Geometry: see drawing. Coordinates: mm, zero at the bounding-box minimum. Coordinates: 2 decimals unless noted, no trailing zeros. Order: outer loops, then holes, each group sorted by start corner. A loop starts at its lowest first (then second) coordinate and runs counter-clockwise, first axis right, second up. Notation, with made-up numbers: (5.5, -5) -> (62.5, -5) arc R23 cw to (62.5, 17) -> close; hole circle Ø7 at (-35, 70). An arc over 180 degrees is marked (long way). Use one line per item in the form item = value.
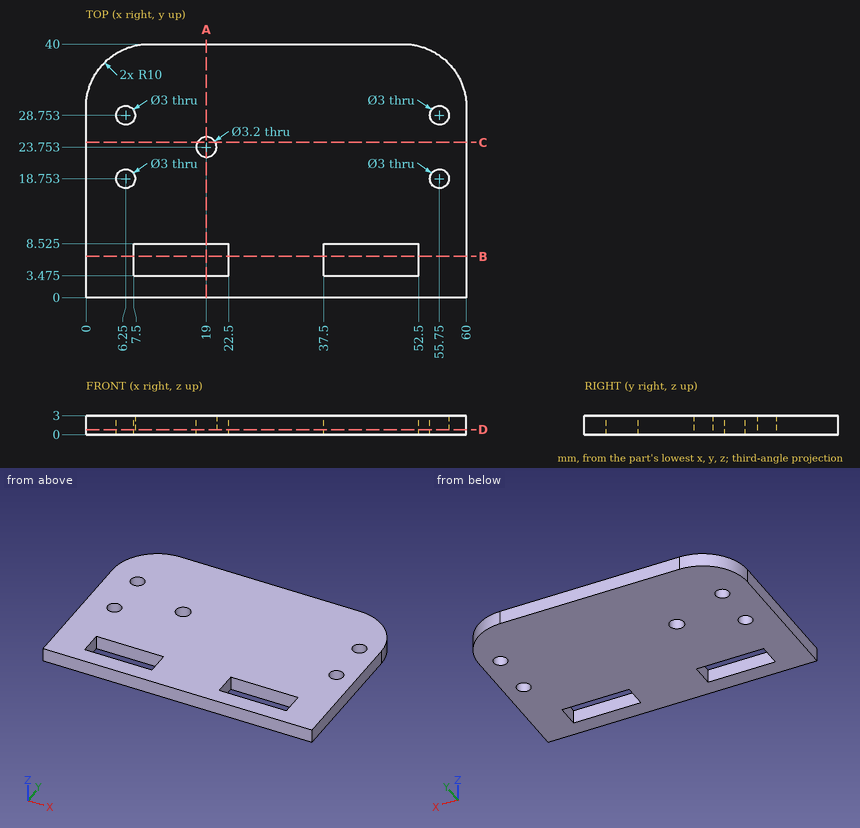
1) Section B-B, the plane y = 6.5. Output: boundary loops of the cut face in (x, z), and give its area (3 significant figures).
Results found:
outline = (0, 0) -> (7.5, 0) -> (7.5, 3) -> (0, 3) -> close; (22.5, 0) -> (37.5, 0) -> (37.5, 3) -> (22.5, 3) -> close; (52.5, 0) -> (60, 0) -> (60, 3) -> (52.5, 3) -> close
area = 90.0 mm2
2) Section C-C, the plane y = 24.5. Output: boundary loops of the cut face in (x, z) (3 decimals).
Results found:
outline = (0, 0) -> (17.585, 0) -> (17.585, 3) -> (0, 3) -> close; (20.415, 0) -> (60, 0) -> (60, 3) -> (20.415, 3) -> close
3) Contact query for flat-ended pins moving along their axis: P1, Ø0.9, axis at x = 17, z = 1, coming from the -Y side; P2, Ø2.5, axis at x = 55.75, y = 18.75, coming from the -Z side. Output: stop coordinate, or through.
Results found:
P1 = 0
P2 = through
4) Section A-A, the plane x = 19. Output: boundary loops of the cut face in (y, z) (1 decimal).
Results found:
outline = (0, 0) -> (3.5, 0) -> (3.5, 3) -> (0, 3) -> close; (8.5, 0) -> (22.2, 0) -> (22.2, 3) -> (8.5, 3) -> close; (25.4, 0) -> (40, 0) -> (40, 3) -> (25.4, 3) -> close
5) Material intervals for probe 1 along X at (y, z) = (8, 1.55); probe 2 along Y at (x, z) = (19, 0.85) (1 decimal); probe 3 along Y at (x, z) = (12, 1.9) (3 decimals), sorted ascending. Write a range as from..to.
Results found:
probe_1 = 0..7.5, 22.5..37.5, 52.5..60
probe_2 = 0..3.5, 8.5..22.2, 25.4..40
probe_3 = 0..3.475, 8.525..40
6) Section D-D, the plane z = 0.8. Give the number of separate pieces and of enclosed holes in the cut face, and give its area (3 significant figures).
Results found:
separate_pieces = 1
enclosed_holes = 7
area = 2,170 mm2
